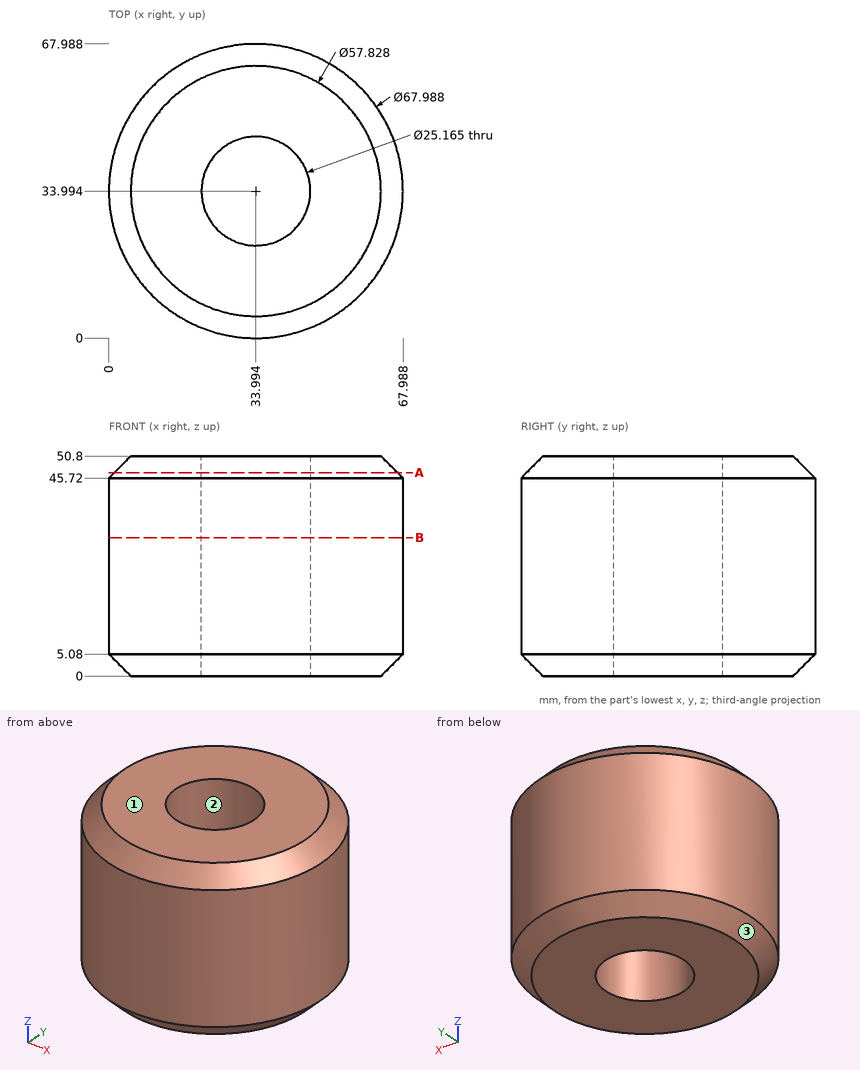
Geometry: see drawing. Coordinates: mm, zero at the bounding-box minimum. Give positions to 0.01 mm unless a question says otherwise; leave off trailing zeros. Order: outer loops, then holes, each group sorted by start corner. A loop starts at its lowest first (then second) coordinate and runs counter-clockwise, first axis right, second up.
1. Cut plane B-B (z = 32). Return loops of the section in (x, y) (1 decimal).
Computed:
outline: circle Ø68 at (34, 34); hole circle Ø25.2 at (34, 34)
2. Line query: probe 1 along X at (y, z) = (34, 18); probe 2 along X at (y, z) = (42, 44.5) (1 decimal). Output: solid intervals per line, ascending.
Computed:
probe 1: x = 0 to 21.41, 46.58 to 67.99
probe 2: x = 1 to 24.3, 43.7 to 67
3. Pin query (flat end, axial travel): pin 1 Ø1 at (y, z) = (11, 38.5) entering from -X (1 decimal); pin 2 Ø1.5 at (x, z) = (12.5, 9) entering from +Y (1 decimal); pin 3 Ø1.5 at (y, z) = (47, 21.5) entering from +X. Return the tip coordinate at first contact, or that it passes through.
Computed:
pin 1: stops at x = 8.5
pin 2: stops at y = 60.9
pin 3: stops at x = 65.7
4. Draft query along X for the marked faces 1, 2 and 3. Return one class per face: released by +X, released by -X, zero draft, split by the parting line, or undercut.
Computed:
face 1: zero draft
face 2: undercut
face 3: split by the parting line
5. Cut plane A-A (z = 47). Return loops of the section in (x, y) (1 decimal).
Computed:
outline: circle Ø65.4 at (34, 34); hole circle Ø25.2 at (34, 34)
